```python
from build123d import *

# Parameters (mm, degrees)
BOSS_EXTRUDE1_DEPTH = 30.607
SKETCH2_R           = 1.2954
CUT_EXTRUDE1_DEPTH  = 52.838718059


with BuildPart() as part:
    # Sketch1 → Boss-Extrude1 (new body)
    with BuildSketch(Plane.XY):
        Polygon((-4.7625, 0), (5.08, 0), (5.08, -41.529), (-4.7625, -41.529), (-4.7625, -36.7665), (0.3175, -36.7665), (0.3175, -4.7625), (-4.7625, -4.7625), align=None)
    extrude(amount=BOSS_EXTRUDE1_DEPTH)

    # Sketch2 → Cut-Extrude1 (cut, through all)
    with BuildSketch(Plane(origin=(0, 0, 0), x_dir=(1, 0, 0), z_dir=(0, 1, 0))):
        with Locations(Location((-2.1717, -27.305, 0), (0, 0, 270))):
            Circle(SKETCH2_R)
        with Locations(Location((-2.1717, -19.304, 0), (0, 0, 270))):
            Circle(SKETCH2_R)
        with Locations(Location((-2.1717, -3.302, 0), (0, 0, 90))):
            Circle(SKETCH2_R)
        with Locations(Location((-2.1717, -11.303, 0), (0, 0, 90))):
            Circle(SKETCH2_R)
    extrude(amount=-CUT_EXTRUDE1_DEPTH, mode=Mode.SUBTRACT)


solid = part.part
```
The listing builds one solid part. Answer for the finished solid, in the listing's coordinates (mm). A direction names the side the tool comes from. Give positions to 0.01 mm unless a question says otherwise; leave off trailing zeros. Write each loop counter-clockwise with the first axis right and the second up, starting at its lowest first coordinate (ties: lowest second). Pieces come first, ordered by that corner, then holes. Notation, with made-up numbers: M -16.75,18 L -7.75,18 A19 ccw -7.75,37 Z; hole C 57.5,4 d9. An arc over 180 degrees is marked long. Write each question's results on one line, items separated by ' | '.
Q1. For a pull along X with two mould halves and no side action, classify faces 1 (the cylindrical face through (-1.676, -39.114, 10.106)), 2 (the flat face through (0.318, -21, 15)), 3 (the flat face through (5.08, -20, 15)), 4 (the flat face through (-2, -4.762, 15)) as released by +X, released by -X, zero draft, split by the parting line, or undercut.
Output values:
face 1: undercut | face 2: released by -X | face 3: released by +X | face 4: zero draft
Q2. A flat-ended cylindrical pin translates along its axis: P1, Ø1.5, axis at y = -18.5, z = 16.5, coming from the -X side. Find the tip coordinate at first contact, or state that the pin passes through.
Output values:
P1: x = 0.32
Q3. A tool of negligible diameter and unlimited length cuts with its end or side. For faces 5 (the flat face through (2, -20, 30.607)), 6 (the flat face through (-2, -36.766, 15)), from which of +Z, -Z, +X, -X, +Y, -Y can it reach the whole face along a straight path? Write none if from no direction.
Output values:
face 5: +Z, +X, -X, +Y, -Y | face 6: +Z, -Z, -X
Q4. Consider L1, parallel to X at y = -8.5, z = 15.5; L2, parallel to Y at x = -1.25, z = 6.5; L3, parallel to X at y = -37, z = 11.5. Determine where each line is inside the solid, lowest interval first. Write a range as from..to.
Output values:
L1: 0.32..5.08 | L2: -41.53..-36.77, -4.76..0 | L3: -4.76..-3.45, -0.89..5.08
Q5. Section A-A, the plane z = 8 is taken. Write down the section's boundary in (x, y), then the cut area to 3 significant figures.
Output values:
outline: M -4.76,-41.53 L 5.08,-41.53 L 5.08,0 L -4.76,0 L -4.76,-4.76 L 0.32,-4.76 L 0.32,-36.77 L -4.76,-36.77 Z | area: 246 mm2
Q6. Section B-B, the plane z = 19 is taken. Write down the section's boundary in (x, y), then the cut area to 3 significant figures.
Output values:
outline: M -4.76,-41.53 L -3.43,-41.53 L -3.43,-36.77 L -4.76,-36.77 Z; M -4.76,-4.76 L -3.43,-4.76 L -3.43,0 L -4.76,0 Z; M -0.91,-41.53 L 5.08,-41.53 L 5.08,0 L -0.91,0 L -0.91,-4.76 L 0.32,-4.76 L 0.32,-36.77 L -0.91,-36.77 Z | area: 222 mm2
Q7. Section C-C, the plane y = -23 is taken. Write down the section's boundary in (x, z), then the cut area to 3 significant figures.
Output values:
outline: M 0.32,0 L 5.08,0 L 5.08,30.61 L 0.32,30.61 Z | area: 146 mm2
